```python
from build123d import *
from OCP.BRepFilletAPI import BRepFilletAPI_MakeChamfer

# Parameters (mm, degrees)
SKETCH_1_R       = 3
SKETCH_1_R_2     = 4
SKETCH_1_R_3     = 1.25
SKETCH_1_R_4     = 1.5
EXTRUDE_1_DEPTH  = 2
CHAMFER_1_SIZE   = 1.5
CHAMFER_1_SIZE_2 = 2


with BuildPart() as part:
    # 草图1 → 凸台-拉伸1 (new body)
    # profile 1 of 3: a face of its own
    with BuildSketch(Plane.XY):
        with BuildLine():
            ThreePointArc((-105.718905787, 7.244728588), (-102.151651286, 4.140596435), (-97.556989056, 3.022553461))
            Line((-97.556989056, 3.022553461), (-0.921282848, 3.022639283))
            Line((-0.921282848, 3.022639283), (95.714423361, 3.022750547))
            ThreePointArc((95.714423361, 3.022750547), (100.30908331, 4.140802892), (103.87633148, 7.24494232))
            ThreePointArc((103.87633148, 7.24494232), (126.57834594, -0.028036342), (103.817957269, -7.116222762))
            ThreePointArc((103.817957269, -7.116222762), (100.989655875, -4.398243929), (97.333501186, -2.977247589))
            Line((97.333501186, -2.977247589), (-0.921276729, -2.977360717))
            Line((-0.921276729, -2.977360717), (-99.176054645, -2.977447977))
            ThreePointArc((-99.176054645, -2.977447977), (-102.832206436, -4.398451774), (-105.660502287, -7.116436375))
            ThreePointArc((-105.660502287, -7.116436375), (-128.420905414, -0.028296374), (-105.718905787, 7.244728588))
        make_face()
        with Locations((-121.57813209, -5.634211545)):
            Circle(SKETCH_1_R, mode=Mode.SUBTRACT)
        with Locations((-115.921163949, 0.022537151)):
            Circle(SKETCH_1_R_2, mode=Mode.SUBTRACT)
        with Locations((119.735576409, -5.634211545)):
            Circle(SKETCH_1_R, mode=Mode.SUBTRACT)
        with Locations((112.202284082, -6.980319536)):
            Circle(SKETCH_1_R_3, mode=Mode.SUBTRACT)
        with Locations((114.078604371, 0.022771691)):
            Circle(SKETCH_1_R_2, mode=Mode.SUBTRACT)
        with Locations((-110.794753677, 5.149166868)):
            Circle(SKETCH_1_R_3, mode=Mode.SUBTRACT)
        with Locations((-122.924240081, 1.899080781)):
            Circle(SKETCH_1_R_3, mode=Mode.SUBTRACT)
        with Locations((121.0816844, 1.899080781)):
            Circle(SKETCH_1_R_3, mode=Mode.SUBTRACT)
        with Locations((-114.044839764, -6.980319536)):
            Circle(SKETCH_1_R_3, mode=Mode.SUBTRACT)
        with Locations((108.952197996, 5.149166868)):
            Circle(SKETCH_1_R_3, mode=Mode.SUBTRACT)
    # profile 2 of 3: a face of its own
    with BuildSketch(Plane.XY):
        with Locations((-121.57813209, -5.634211545)):
            Circle(SKETCH_1_R)
        with Locations((-121.57813209, -5.634211545)):
            Circle(SKETCH_1_R_4, mode=Mode.SUBTRACT)
    # profile 3 of 3: a face of its own
    with BuildSketch(Plane.XY):
        with Locations((119.735576409, -5.634211545)):
            Circle(SKETCH_1_R)
        with Locations((119.735576409, -5.634211545)):
            Circle(SKETCH_1_R_4, mode=Mode.SUBTRACT)
    extrude(amount=EXTRUDE_1_DEPTH)

    # 倒角1
    chamfer_1_edges_1 = [part.edges().sort_by_distance(p)[0] for p in [
        (118.235576409, -5.634211545, 2),
    ]]
    chamfer_1_side_1 = [part.faces().sort_by_distance(p)[0] for p in [
        (118.205576409, -5.634211545, 2),
    ]]
    chamfer_1_edges_2 = [part.edges().sort_by_distance(p)[0] for p in [
        (-123.07813209, -5.634211545, 2),
    ]]
    chamfer_1_side_2 = [part.faces().sort_by_distance(p)[0] for p in [
        (-123.10813209, -5.634211545, 2),
    ]]
    chamfer_1 = BRepFilletAPI_MakeChamfer(part.part.solid().wrapped)
    for e in chamfer_1_edges_1:
        chamfer_1.Add(CHAMFER_1_SIZE - 0.0001, CHAMFER_1_SIZE_2 - 0.0001, e.wrapped, chamfer_1_side_1[0].wrapped)
    for e in chamfer_1_edges_2:
        chamfer_1.Add(CHAMFER_1_SIZE - 0.0001, CHAMFER_1_SIZE_2 - 0.0001, e.wrapped, chamfer_1_side_2[0].wrapped)
    add(Compound.cast(chamfer_1.Shape()), mode=Mode.REPLACE)  # a hair under: the kernel refuses the full size


solid = part.part
```
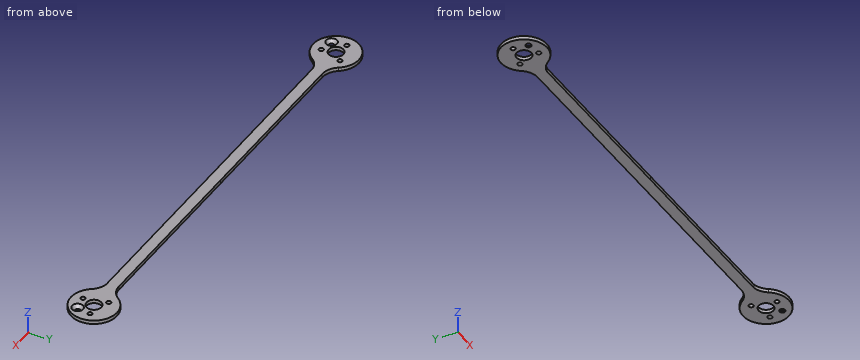
Input: part model. Units: mm. Frame: model coordinates. Round coordinates to 2 decimals unless told otherwise and drop trailing zeros. Order: outer loops, then holes, each group sorted by start corner. A loop starts at its lowest first (then second) coordinate and runs counter-clockwise, first axis right, second up. Notation, with made-up numbers: (27, -37) - (54, -37) arc R25 cw to (54, 1) - close; hole circle Ø6 at (-5, 76). An arc over 180 degrees is marked (long way). Answer in a Markdown table with one row per item.
Item 1: Line query: line 1 (X direction, y = -6.5, z = 0.85); line 2 (X direction, y = 4.75, z = 0.2); line 3 (X direction, y = 2.5, z = 1). Output: solid intervals per line, ascending.
Model answer:
| item | result |
|---|---|
| line 1 | x = -126.58 to -123.53, -119.62 to -115.2, -112.89 to -105.2, 103.35 to 111.05, 113.36 to 117.78, 121.69 to 124.74 |
| line 2 | x = -127.49 to -111.98, -109.61 to -103.18, 101.33 to 107.77, 110.14 to 125.65 |
| line 3 | x = -128.17 to -124.02, -121.83 to -119.06, -112.78 to 110.94, 117.22 to 119.99, 122.18 to 126.33 |
Item 2: Section query B-B (x = 17). Return the cut outline in (y, z), then the cut area to 3 significant figures.
Model answer:
| item | result |
|---|---|
| outline | (-2.98, 0) - (3.02, 0) - (3.02, 2) - (-2.98, 2) - close |
| area | 12.0 mm² |
Item 3: Pin query (flat end, axial travel): pin 1 (5 mm diameter, centred on x = 119.74, y = -5.63, fed in from -Z); pin 2 (2 mm diameter, centred on x = 121.08, y = 1.9, fed in from -Z); pin 3 (1 mm diameter, centred on y = -3, z = 1.5, fed in from +X); pin 4 (1 mm diameter, centred on x = -68.5, z = 1.5, fed in from -Y). Return the tip coordinate at first contact, or that it passes through.
Model answer:
| item | result |
|---|---|
| pin 1 | stops at z = 0 |
| pin 2 | passes through |
| pin 3 | stops at x = 126.32 |
| pin 4 | stops at y = -2.98 |
Item 4: Section query A-A (z = 0.6). Give the number of separate pieces and of enclosed holes in the cut face, then the cut area to 3 significant figures.
Model answer:
| item | result |
|---|---|
| separate pieces | 1 |
| enclosed holes | 10 |
| area | 2,080 mm² |
